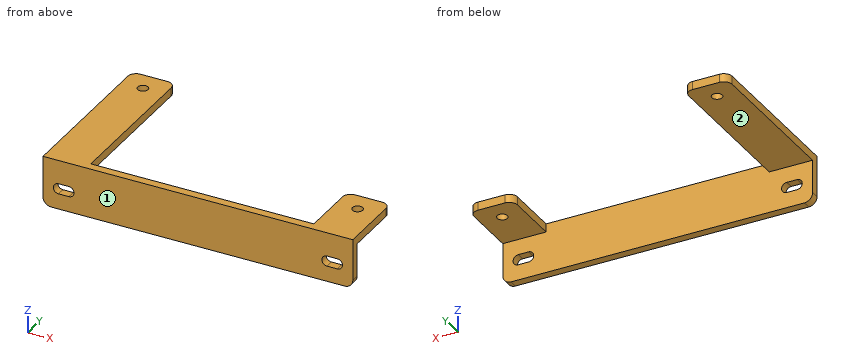
from build123d import *

# Parameters (mm, degrees)
SKETCH1_W           = 150
SKETCH1_H           = 20
BOSS_EXTRUDE1_DEPTH = 4
SKETCH2_W           = 21
SKETCH2_H           = 76.95216022
SKETCH2_R           = 2.5
SKETCH2_H_2         = 4
SKETCH2_W_2         = 108
SKETCH2_H_3         = 30
BOSS_EXTRUDE2_DEPTH = 4
FILLET1_R           = 4


with BuildPart() as part:
    # Sketch1 → Boss-Extrude1 (new body)
    with BuildSketch(Plane(origin=(0, 0, 0), x_dir=(1, 0, 0), z_dir=(0, 1, 0))):
        Rectangle(SKETCH1_W, SKETCH1_H)
        with BuildLine():
            Line((-67.5, 2.5), (-62.5, 2.5))
            ThreePointArc((-62.5, 2.5), (-60, 0), (-62.5, -2.5))
            Line((-62.5, -2.5), (-67.5, -2.5))
            ThreePointArc((-67.5, -2.5), (-70, 0), (-67.5, 2.5))
        make_face(mode=Mode.SUBTRACT)
        with BuildLine():
            Line((62.5, 2.5), (67.5, 2.5))
            ThreePointArc((67.5, 2.5), (70, 0), (67.5, -2.5))
            Line((67.5, -2.5), (62.5, -2.5))
            ThreePointArc((62.5, -2.5), (60, 0), (62.5, 2.5))
        make_face(mode=Mode.SUBTRACT)
    extrude(amount=BOSS_EXTRUDE1_DEPTH)

    # Sketch2 → Boss-Extrude2 (add)
    # profile 1 of 5: a face of its own
    with BuildSketch(Plane.XY.offset(10)):
        with Locations((-64.5, 42.47608011)):
            Rectangle(SKETCH2_W, SKETCH2_H)
        with Locations((-64.5, 70.95216022)):
            Circle(SKETCH2_R, mode=Mode.SUBTRACT)
    # profile 2 of 5: a face of its own
    with BuildSketch(Plane.XY.offset(10)):
        with Locations((-64.5, 2)):
            Rectangle(SKETCH2_W, SKETCH2_H_2)
    # profile 3 of 5: a face of its own
    with BuildSketch(Plane.XY.offset(10)):
        with Locations((0, 2)):
            Rectangle(SKETCH2_W_2, SKETCH2_H_2)
    # profile 4 of 5: a face of its own
    with BuildSketch(Plane.XY.offset(10)):
        with Locations((64.5, 2)):
            Rectangle(SKETCH2_W, SKETCH2_H_2)
    # profile 5 of 5: a face of its own
    with BuildSketch(Plane.XY.offset(10)):
        with Locations((64.5, 19)):
            Rectangle(SKETCH2_W, SKETCH2_H_3)
        with Locations((64.5, 24)):
            Circle(SKETCH2_R, mode=Mode.SUBTRACT)
    extrude(amount=BOSS_EXTRUDE2_DEPTH)

    # Fillet1
    fillet1_edges = [part.edges().sort_by_distance(p)[0] for p in [
        (-75, 80.95216022, 12),
        (75, 34, 12),
        (54, 34, 12),
        (-54, 80.95216022, 12),
        (-75, 2, -10),
        (75, 2, -10),
    ]]
    fillet(fillet1_edges, radius=FILLET1_R)


solid = part.part
Read the model definition and answer for the solid it produces. Units are mm, in the model's axes. Face numbers are marked on the shaded views. A direction names the side the tool comes from. Give positions to 0.01 mm unless a question says otherwise; leave off trailing zeros. Loops run counter-clockwise (first coordinate to the right, second up) from the corner with the lowest first, then second, coordinate; pieces in that order, holes last. Notation, with made-up numbers: (-17, -8.5) -> (29, -8.5) arc R20 cw to (29, 22.5) -> close; hole circle Ø9 at (-18, 44). An arc over 180 degrees is marked (long way). Use a Markdown table: item, result.
Q1. Section C-C, the plane z = 0 is taken. Determine the outline of the cut face in (x, y), then the cut area to 3 significant figures.
Solved:
| item | result |
|---|---|
| outline | (-75, 0) -> (-70, 0) -> (-70, 4) -> (-75, 4) -> close; (-60, 0) -> (60, 0) -> (60, 4) -> (-60, 4) -> close; (70, 0) -> (75, 0) -> (75, 4) -> (70, 4) -> close |
| area | 520 mm^2 |
Q2. Section A-A, the plane y = 7 is taken. Determine the outline of the cut face in (x, z).
Solved:
| item | result |
|---|---|
| outline | (-75, 10) -> (-54, 10) -> (-54, 14) -> (-75, 14) -> close; (54, 10) -> (75, 10) -> (75, 14) -> (54, 14) -> close |
Q3. A tool of negligible diameter and unlimited length cuts with its end or side. For the marked faces 1 and 2, from which of +Z, -Z, +X, -X, +Y, -Y can it reach the whole face along a straight path? Write none if from no direction.
Solved:
| item | result |
|---|---|
| face 1 | +Z, -Z, +X, -X, -Y |
| face 2 | -Z, +X, -X, +Y |
Q4. Section D-D, the plane y = 24 is taken. Determine the outline of the cut face in (x, z).
Solved:
| item | result |
|---|---|
| outline | (-75, 10) -> (-54, 10) -> (-54, 14) -> (-75, 14) -> close; (54, 10) -> (62, 10) -> (62, 14) -> (54, 14) -> close; (67, 10) -> (75, 10) -> (75, 14) -> (67, 14) -> close |
Q5. Each of these flat-tipped pins is pushed along its axis until it touches: pin 1 (3 mm diameter, centred on y = 36, z = 12, fed in from +X); pin 2 (3 mm diameter, centred on x = 61.5, z = 11, fed in from +Y); pin 3 (1.5 mm diameter, centred on x = -25.5, z = 9, fed in from +Y). Where does it stop, or does it pass through?
Solved:
| item | result |
|---|---|
| pin 1 | stops at x = -54 |
| pin 2 | stops at y = 34 |
| pin 3 | stops at y = 4 |
Q6. Find the intervals of material crossed by line 1 along Y through (x, z) = (64.5, 12.15); line 2 along Y through (x, z) = (-64.5, 11.55); line 3 along X through (y, z) = (29.5, 12.75), in increasing order.
Solved:
| item | result |
|---|---|
| line 1 | y = 0 to 21.5, 26.5 to 34 |
| line 2 | y = 0 to 68.45, 73.45 to 80.95 |
| line 3 | x = -75 to -54, 54 to 75 |
Q7. Section B-B, the plane x = -64.5 is taken. Determine the outline of the cut face in (y, z), then the cut area to 3 significant figures.
Solved:
| item | result |
|---|---|
| outline | (0, -10) -> (4, -10) -> (4, -2.5) -> (0, -2.5) -> close; (0, 2.5) -> (4, 2.5) -> (4, 10) -> (68.45, 10) -> (68.45, 14) -> (0, 14) -> close; (73.45, 10) -> (80.95, 10) -> (80.95, 14) -> (73.45, 14) -> close |
| area | 364 mm^2 |
